```python
from build123d import *

# Parameters (mm, degrees)
SKETCH1_R           = 15
SKETCH1_R_2         = 9
BOSS_EXTRUDE1_DEPTH = 7
CIRPATTERN1_COUNT   = 6
CHAMFER1_SIZE       = 0.5


with BuildPart() as part:
    # Sketch1 → Boss-Extrude1 (new body)
    with BuildSketch(Plane(origin=(0, 0, 0), x_dir=(0, 0, -1), z_dir=(1, 0, 0))):
        Circle(SKETCH1_R)
        Circle(SKETCH1_R_2, mode=Mode.SUBTRACT)
    extrude(amount=BOSS_EXTRUDE1_DEPTH)

    # Sketch3 → Ø4.0mm Dowel Hole1 (revolve, cut)
    with BuildSketch(Plane(origin=(7, 12, 0), x_dir=(0, 0, -1), z_dir=(0, 1, 0))):
        Polygon((0, 0), (0, 51.201721238), (2, 50), (2, 0), align=None)
    f_4_0mm_dowel_hole1 = revolve(axis=Axis((13.35, 12, 0), (-1, 0, 0)), mode=Mode.SUBTRACT)

    # CirPattern1: Ø4.0mm Dowel Hole1 ×6 about axis
    cirpattern1_axis = Axis((0, 0, 0), (1, 0, 0))
    for i in range(1, CIRPATTERN1_COUNT):
        add(f_4_0mm_dowel_hole1.rotate(cirpattern1_axis, i * 360 / CIRPATTERN1_COUNT), mode=Mode.SUBTRACT)

    # Chamfer1
    chamfer1_edges = [part.edges().sort_by_distance(p)[0] for p in [
        (7, 0, 15),
    ]]
    chamfer(chamfer1_edges, length=CHAMFER1_SIZE)


solid = part.part
```
Could you check a few things on this model? Use its own coordinates, in mm. Coordinates: 2 decimals unless noted, no trailing zeros. Loops run counter-clockwise (first coordinate to the right, second up) from the corner with the lowest first, then second, coordinate; pieces in that order, holes last. Notation, with made-up numbers: M 88,-27.75 L 107,-27.75 A24 ccw 107,-17.75 Z; hole C 83.25,-22.5 d1. An arc over 180 degrees is marked long. Put each result on its own line as item: value. Start each with the question number.
(1) Will these pins go through, and if not, where does the flat tip stop? P1, Ø3, axis at x = 3.5, y = -11.5, coming from the -Z side; P2, Ø4, axis at x = 3.5, z = 4.5, coming from the -Y side.
(2) Suppose I cut it at B-B on x = 3.25. Please give me the cut outline in (y, z).
(3) Thinking about a two-plate mould opening in Z: for faces 1 (the face through (3.204, 0.66, 14.985)), 2 (the face through (3.549, 7.983, -10.653)), 3 (the face through (7, -6, 7)), which applies, pulls with the +Z half, pulls with the -Z half, needs draft (parallel to the pull), parting line crosses it, or undercut?
(4) I need wall thicknesses on line 1 (Y direction, x = 4, z = 0); line 2 (Z direction, x = 2.75, y = 6.25); line 3 (Z direction, x = 1.5, y = -12). Which ranges of each line are inside material? Lowest first, please. Write a range as from..to.
(5) Suppose I cut it at A-A on z = 0. Please give me the cut outline in (x, y), then the cut area to 4 significant figures.
(6) Suppose I cut it at C-C on y = 6. Count the separate pieces of the cut face and the enclosed holes in it, then the cut area to 3 significant figures.
Solutions:
1. P1: stops at z = -11.18
1. P2: stops at y = -14.79
2. outline: C 0,0 d30; hole C -12,0 d4; hole C 0,0 d18; hole C -6,-10.39 d4; hole C -6,10.39 d4; hole C 6,-10.39 d4; hole C 6,10.39 d4; hole C 12,0 d4
3. face 1: parting line crosses it
3. face 2: undercut
3. face 3: needs draft
4. line 1: y = -15..-14, -10..-9, 9..10, 14..15
4. line 2: z = -13.64..-12.38, -8.41..-6.48, 6.48..8.41, 12.38..13.64
4. line 3: z = -9..-2, 2..9
5. outline: M 0,-15 L 6.5,-15 L 7,-14.5 L 7,-14 L 0,-14 Z; M 0,-10 L 7,-10 L 7,-9 L 0,-9 Z; M 0,9 L 7,9 L 7,10 L 0,10 Z; M 0,14 L 7,14 L 7,14.5 L 6.5,15 L 0,15 Z
5. area: 27.75 mm2
6. separate pieces: 4
6. enclosed holes: 0
6. area: 42.3 mm2
